Geometry check sheet. Reference: the model listing, model coordinates, mm. A direction names the side the tool comes from. Coordinates: 2 decimals unless noted, no trailing zeros. Loops run counter-clockwise (first coordinate to the right, second up) from the corner with the lowest first, then second, coordinate; pieces in that order, holes last.
from build123d import *

# Parameters (mm, degrees)
SKETCH003_R     = 1
PAD_DEPTH       = 1.2
PAD014_DEPTH    = 1.2713
POCKET004_DEPTH = 7.5


with BuildPart() as part:
    # Sketch003 → Pad (new body)
    with BuildSketch(Plane.XY):
        Polygon((-19.62132, 14.62132), (-15.37868, 14.62132), (19.62132, 14.62132), (19.62132, 10.37868), (0, 10.37868), (-3, 8), (-3, 0), (0, -3), (5, -3), (19.62132, -10.37868), (19.62132, -14.62132), (-19.62132, -14.62132), align=None)
        with Locations((-17.5, 12.5)):
            Circle(SKETCH003_R, mode=Mode.SUBTRACT)
        with Locations((-17.5, -12.5)):
            Circle(SKETCH003_R, mode=Mode.SUBTRACT)
        with Locations((17.5, -12.5)):
            Circle(SKETCH003_R, mode=Mode.SUBTRACT)
        with Locations((17.5, 12.5)):
            Circle(SKETCH003_R, mode=Mode.SUBTRACT)
    extrude(amount=-PAD_DEPTH)

    # Sketch019 (on DatumPlane) → Pad014 (join)
    with BuildSketch(Plane.XZ.offset(14.6213)):
        Polygon((-10, 0), (-7.5, 1.6), (7.5, 1.6), (10, 0), align=None)
    pad014 = extrude(amount=-PAD014_DEPTH)

    # Sketch → Pocket004 (cut, symmetric)
    with BuildSketch(Plane.YZ):
        with BuildLine():
            ThreePointArc((-13.35, -0.209228), (-13.246442, -0.411848), (-13.021562, -0.446604))
            Line((-13.021562, -0.446604), (-11.67, 0))
            Line((-13.35, 0), (-11.67, 0))
            Line((-13.35, -0.209228), (-13.35, 0))
        make_face()
    pocket004 = extrude(amount=POCKET004_DEPTH, both=True, mode=Mode.SUBTRACT)

    # Mirrored: Pad014, Pocket004 across XZ
    add(pad014.mirror(Plane.XZ))
    add(pocket004.mirror(Plane.XZ), mode=Mode.SUBTRACT)


solid = part.part
1) Access from +Z, -Z, +X, -X, +Y, -Y to the whole of each face (thin tool, end or side, straight path). Record for faces 4 (the flat face through (0.11, 12.36, -0.23)), 5 (the flat face through (12.21, -6.64, -0.59)), 6 (the flat face through (0, -14.621, 1)).
Data:
face 4: +Z
face 5: +Z, -Z, +X
face 6: +Z, -Z, +X, -X, -Y
2) Section check A-A on x = -17.5. Record the cut outline in (y, z), and give its area (3 significant figures).
Data:
outline: (-14.62, -1.2) - (-13.5, -1.2) - (-13.5, 0) - (-14.62, 0) - close; (-11.5, -1.2) - (11.5, -1.2) - (11.5, 0) - (-11.5, 0) - close; (13.5, -1.2) - (14.62, -1.2) - (14.62, 0) - (13.5, 0) - close
area: 30.3 mm2
3) Depth check by flat-ended pin: pin 1 (6 mm diameter, centred on x = -2.5, y = 7, fed in from +Z); pin 2 (1 mm diameter, centred on y = 5.5, z = -0.5, fed in from +X). Enter the tip coordinate at first touch or a pass-through.
Data:
pin 1: stops at z = 0
pin 2: stops at x = -3
4) Section check B-B on y = -12.5. Record the cut outline in (x, z), and give its area (3 significant figures).
Data:
outline: (-19.62, -1.2) - (-18.5, -1.2) - (-18.5, 0) - (-19.62, 0) - close; (-16.5, -1.2) - (16.5, -1.2) - (16.5, 0) - (7.5, 0) - (7.5, -0.27) - (-7.5, -0.27) - (-7.5, 0) - (-16.5, 0) - close; (18.5, -1.2) - (19.62, -1.2) - (19.62, 0) - (18.5, 0) - close
area: 38.2 mm2
5) Mould release check, pull along X, two halves, no side actions. Record for faces 1 (the flat face through (-4, 0, 0)), 2 (the flat face through (0.11, -12.36, -0.23)), 3 (the flat face through (-2, -1, -1)): +X half, -X half, draft (parallel to the pull), parting line (faces both ways), or undercut.
Data:
face 1: draft
face 2: undercut
face 3: +X half
6) Section check C-C on z = 0.7. Record the cut outline in (x, y).
Data:
outline: (-8.91, -14.62) - (8.91, -14.62) - (8.91, -13.35) - (-8.91, -13.35) - close; (-8.91, 13.35) - (8.91, 13.35) - (8.91, 14.62) - (-8.91, 14.62) - close
7) Material ranges on probe 1 along Y at (x, z) = (-17.5, -0.15); probe 2 along Y at (x, z) = (7, 0.2); probe 3 along Y at (x, z) = (17.5, -0.4), recorded low to high.
Data:
probe 1: y = -14.62 to -13.5, -11.5 to 11.5, 13.5 to 14.62
probe 2: y = -14.62 to -13.35, 13.35 to 14.62
probe 3: y = -14.62 to -13.5, -11.5 to -9.31, 10.38 to 11.5, 13.5 to 14.62
